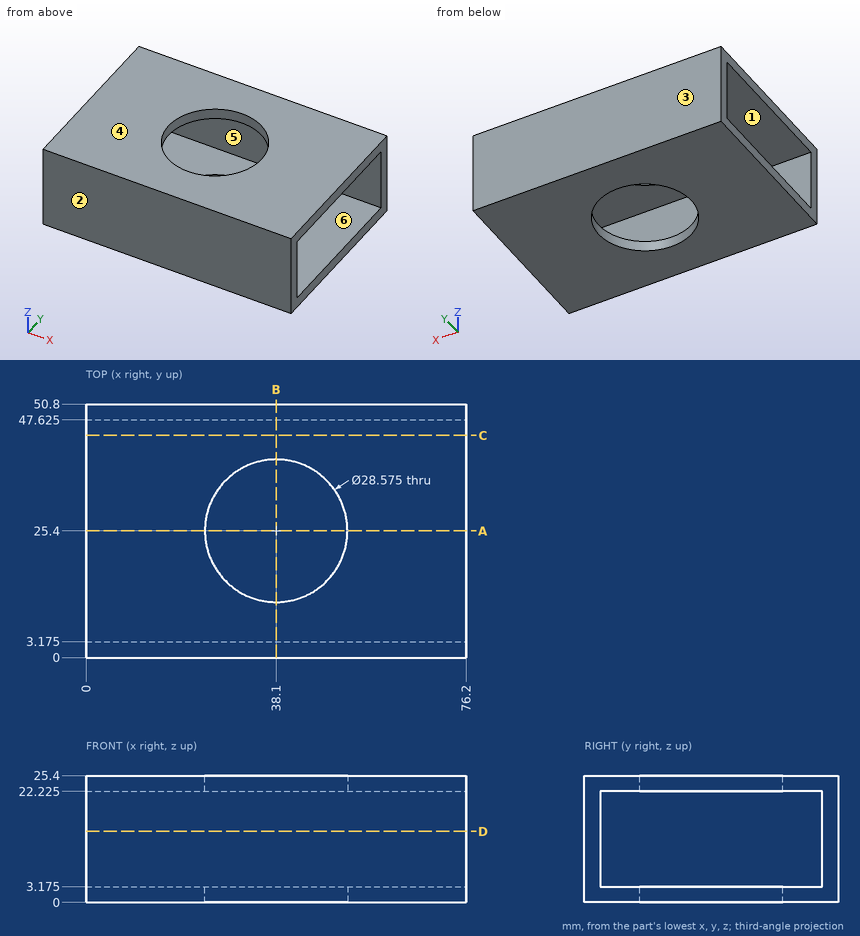
Geometry check sheet. Reference: drawing and pictorial views, mm from the part's lowest x, y, z. A direction names the side the tool comes from. Round coordinates to 2 decimals unless told otherwise and drop trailing zeros. Order: outer loops, then holes, each group sorted by start corner. A loop starts at its lowest first (then second) coordinate and runs counter-clockwise, first axis right, second up. Notation, with made-up numbers: (25.25, -20.75) - (58.25, -20.75) arc R22 cw to (58.25, 5.25) - close; hole circle Ø8 at (63.5, 21). An arc over 180 degrees is marked (long way). Use a Markdown table: item, result. Add a question column.
1) Set-up check for the marked faces 1 and 2: record each of +Z, -Z, +X, -X, +Y, -Y from which the full face is reachable in a straight line by a thin tool's end or side.
2) Section check A-A (y = 25.4). Record the cut outline in (x, z) (1 decimal), then the cut area to 3 significant figures.
3) Thickness scan on line 1 along Z through (x, y) = (31, 40.5) (3 decimals); line 2 along Y through (x, z) = (43.5, 15.25) (3 decimals); line 3 along Y through (x, z) = (38.1, 1.75). Record the ranges inside material, lowest first.
4) Section check D-D (z = 14.25). Record the cut outline in (x, y) (3 decimals), then the cut area to 3 significant figures.
5) Section check B-B (x = 38.1). Record the cut outline in (y, z) (1 decimal), then the cut area to 3 significant figures.
6) Section check C-C (y = 44.5). Record the cut outline in (x, z) (3 decimals).
7) Mould release check, pull along Y, two halves, no side actions. Record for the marked faces 3, 4, 5 and 6: released by +Y, released by -Y, zero draft, split by the parting line, or undercut.
Established:
| question | item | result |
|---|---|---|
| 1 | face 1 | +X, -X |
| 1 | face 2 | +Z, -Z, +X, -X, -Y |
| 2 | outline | (0, 0) - (23.8, 0) - (23.8, 3.2) - (0, 3.2) - close; (0, 22.2) - (23.8, 22.2) - (23.8, 25.4) - (0, 25.4) - close; (52.4, 0) - (76.2, 0) - (76.2, 3.2) - (52.4, 3.2) - close; (52.4, 22.2) - (76.2, 22.2) - (76.2, 25.4) - (52.4, 25.4) - close |
| 2 | area | 302 mm2 |
| 3 | line 1 | 0 to 3.175, 22.225 to 25.4 |
| 3 | line 2 | 0 to 3.175, 47.625 to 50.8 |
| 3 | line 3 | 0 to 11.11, 39.69 to 50.8 |
| 4 | outline | (0, 0) - (76.2, 0) - (76.2, 3.175) - (0, 3.175) - close; (0, 47.625) - (76.2, 47.625) - (76.2, 50.8) - (0, 50.8) - close |
| 4 | area | 484 mm2 |
| 5 | outline | (0, 0) - (11.1, 0) - (11.1, 3.2) - (3.2, 3.2) - (3.2, 22.2) - (11.1, 22.2) - (11.1, 25.4) - (0, 25.4) - close; (39.7, 0) - (50.8, 0) - (50.8, 25.4) - (39.7, 25.4) - (39.7, 22.2) - (47.6, 22.2) - (47.6, 3.2) - (39.7, 3.2) - close |
| 5 | area | 262 mm2 |
| 6 | outline | (0, 0) - (76.2, 0) - (76.2, 3.175) - (0, 3.175) - close; (0, 22.225) - (76.2, 22.225) - (76.2, 25.4) - (0, 25.4) - close |
| 7 | face 3 | released by +Y |
| 7 | face 4 | zero draft |
| 7 | face 5 | undercut |
| 7 | face 6 | undercut |
